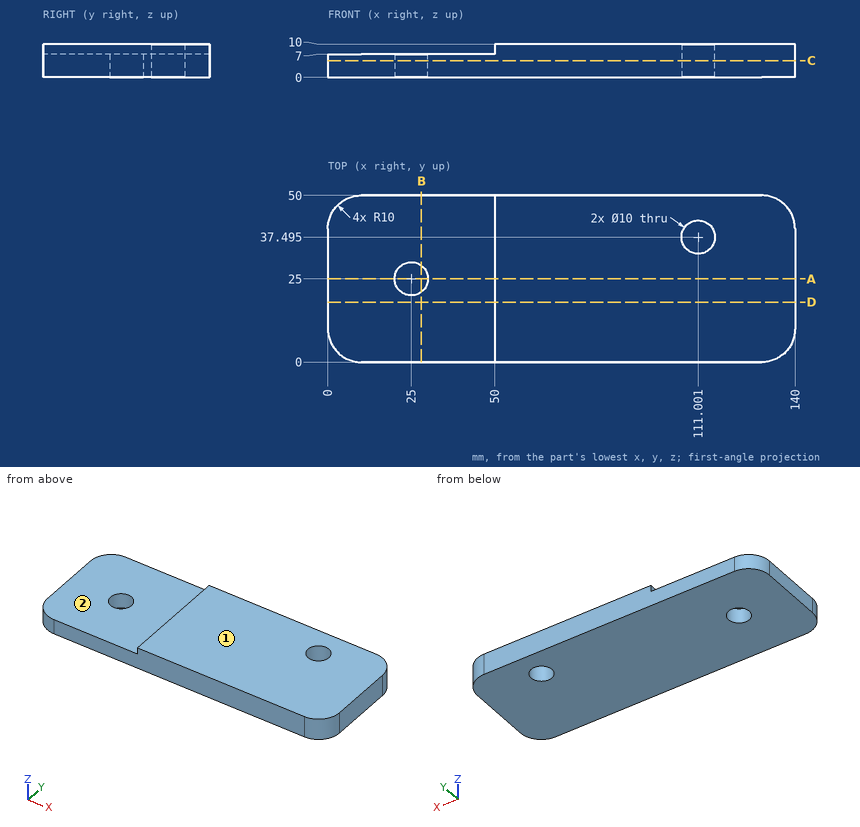
Drawing for the job (mm, zero at the part's lowest x, y, z). A direction names the side the tool comes from. Round coordinates to 2 decimals unless told otherwise and drop trailing zeros. Loops run counter-clockwise (first coordinate to the right, second up) from the corner with the lowest first, then second, coordinate; pieces in that order, holes last. Notation, with made-up numbers: M 64.5,79.25 L 78.5,79.25 A18 ccw 78.5,100.25 Z; hole C 69,49.25 d2. An arc over 180 degrees is marked long. Use a Markdown table: item, result. Add a question column.
(1) Cut at D-D (y = 18). Give the cut face in (x, z), and give its area (3 significant figures).
(2) Which spindle directions (+Z, -Z, +X, -X, +Y, -Y) get a long thin tool onto all of the face, cutting with end or side? Do the marked faces 1 and 2. Say none if no direction does.
(3) Cut at B-B (x = 28). Give the cut face in (y, z), and give its area (3 significant figures).
(4) Drill centre lines: line 1 (Y direction, x = 25, z = 2); line 2 (X direction, y = 25, z = 2); line 3 (Z direction, x = 8, y = 40). Where is each one in solid material? Low to high.
(5) Cut at A-A (y = 25). Give the cut face in (x, z).
(6) Cut at C-C (z = 5). Give the cut face in (x, y) (1 decimal).
(7) Flat gauge pins, fed straight in: pin 1 (1.5 mm diameter, centred on y = 36.5, z = 9, fed in from -X); pin 2 (25 mm diameter, centred on x = 24.5, y = 34, fed in from +Z). Where does each tip first touch, or does it go through?
Geometry says:
| question | item | result |
|---|---|---|
| 1 | outline | M 0,0 L 140,0 L 140,10 L 50,10 L 50,7 L 0,7 Z |
| 1 | area | 1,250 mm² |
| 2 | face 1 | +Z, +X, -X, +Y, -Y |
| 2 | face 2 | +Z, -X, +Y, -Y |
| 3 | outline | M 0,0 L 21,0 L 21,7 L 0,7 Z; M 29,0 L 50,0 L 50,7 L 29,7 Z |
| 3 | area | 294 mm² |
| 4 | line 1 | y = 0 to 20, 30 to 50 |
| 4 | line 2 | x = 0 to 20, 30 to 140 |
| 4 | line 3 | z = 0 to 7 |
| 5 | outline | M 0,0 L 20,0 L 20,7 L 0,7 Z; M 30,0 L 140,0 L 140,10 L 50,10 L 50,7 L 30,7 Z |
| 6 | outline | M 0,10 A10 ccw 10,0 L 130,0 A10 ccw 140,10 L 140,40 A10 ccw 130,50 L 10,50 A10 ccw 0,40 Z; hole C 25,25 d10; hole C 111,37.5 d10 |
| 7 | pin 1 | stops at x = 50 |
| 7 | pin 2 | stops at z = 7 |
